Here's how the part is built. I have some questions about the finished solid (model axes, mm). A direction names the side the tool comes from. Give positions to 0.01 mm unless a question says otherwise; leave off trailing zeros. Loops run counter-clockwise (first coordinate to the right, second up) from the corner with the lowest first, then second, coordinate; pieces in that order, holes last. Notation, with made-up numbers: (59.25, 8.25) -> (96.25, 8.25) arc R9 ccw to (96.25, 18.25) -> close; hole circle Ø11 at (87, 54.5). An arc over 180 degrees is marked (long way). Answer in a Markdown table with one row per item. Add a question column.
Item 1: If we section it at D-D (x = 3.5): Write out the boundary of the cut face in (y, z).
Item 2: For P1, Ø6, axis at x = -4, z = -9.5, coming from the +Y side; P2, Ø2.5, axis at x = -0.5, z = 7, coming from the +Y side (3 decimals); P3, Ø4.5, axis at x = -1.5, z = 3, coming from the -Y side (3 decimals); P4, Ø1.9, axis at x = -0.5, y = -1.5, coming from the +Z side, each with a flat end and sliding along its axis, tell me the tip position at first contact or that it passes through.
Item 3: If we section it at A-A (y = 0): Write out the boundary of the cut face in (x, z) (3 decimals), then the cut area to 3 significant figures.
Item 4: Which directions (+Z, -Z, +X, -X, +Y, -Y) give clear straight access to the entire face, cutting with the end or side of a thin tool? Please do faces 1 (the face through (0, -4, 0)), 2 (the face through (-4.165, 0.051, 5.817)), 3 (the face through (0, -3.175, 6)), 4 (the face through (4.165, -0.051, 5.817)).
Item 5: If we section it at C-C (z = -19): Write out the boundary of the cut face in (x, y), then the cut area to 3 significant figures.
Item 6: If I drill on line 1 (Z direction, x = 2.75, y = -2.5); line 2 (Y direction, x = -1, z = 6) (3 decimals); line 3 (Z direction, x = 0.5, y = 1.5), over which ranges is the centre line in solid material (lowest first)?
Item 7: If we section it at B-B (x = 0): Write out the boundary of the cut face in (y, z) (3 decimals).
```python
from build123d import *

# Parameters (mm, degrees)
SKETCH002_R  = 1.7
PAD002_DEPTH = 5.8
SKETCH003_R  = 1.27
PAD003_DEPTH = 2.9
PAD_DEPTH    = 11.8
SKETCH001_R  = 5.58
PAD001_DEPTH = 32.15


with BuildPart() as metal:
    # Sketch002 → Pad002 (new body)
    with BuildSketch(Plane.XY):
        Circle(SKETCH002_R)
    extrude(amount=PAD002_DEPTH)

    # Sketch003 (on Face3 of Pad002) → Pad003 (join)
    with BuildSketch(Plane.XY.offset(5.8)):
        Circle(SKETCH003_R)
    extrude(amount=PAD003_DEPTH)


with BuildPart() as metal_1:
    # Body001 placement: moved
    add(metal.part.moved(Location((0, 0, 11.8))))


with BuildPart() as obj1:
    # Sketch → Pad (new body)
    with BuildSketch(Plane.XY):
        with BuildLine():
            ThreePointArc((-2.695663, 3.175), (-4.165, 0), (-2.695663, -3.175))
            Line((-2.695663, -3.175), (2.695663, -3.175))
            ThreePointArc((2.695663, -3.175), (4.165, 0), (2.695663, 3.175))
            Line((-2.695663, 3.175), (2.695663, 3.175))
        make_face()
    extrude(amount=PAD_DEPTH)

    # Sketch001 (on Sketch) → Pad001 (join)
    with BuildSketch(Plane.XY):
        Circle(SKETCH001_R)
    extrude(amount=-PAD001_DEPTH)

    # Fusion: union metal
    add(metal_1.part)


solid = obj1.part
```
Recorded:
| question | item | result |
|---|---|---|
| 1 | outline | (-4.35, -32.15) -> (4.35, -32.15) -> (4.35, 0) -> (2.26, 0) -> (2.26, 11.8) -> (-2.26, 11.8) -> (-2.26, 0) -> (-4.35, 0) -> close |
| 2 | P1 | stops at y = 5.49 |
| 2 | P2 | stops at y = 3.175 |
| 2 | P3 | stops at y = -3.175 |
| 2 | P4 | stops at z = 20.5 |
| 3 | outline | (-5.58, -32.15) -> (5.58, -32.15) -> (5.58, 0) -> (4.165, 0) -> (4.165, 11.8) -> (1.7, 11.8) -> (1.7, 17.6) -> (1.27, 17.6) -> (1.27, 20.5) -> (-1.27, 20.5) -> (-1.27, 17.6) -> (-1.7, 17.6) -> (-1.7, 11.8) -> (-4.165, 11.8) -> (-4.165, 0) -> (-5.58, 0) -> close |
| 3 | area | 484 mm^2 |
| 4 | face 1 | +Z |
| 4 | face 2 | +Z, -X |
| 4 | face 3 | +Z, +X, -X, -Y |
| 4 | face 4 | +Z, +X |
| 5 | outline | circle Ø11.16 at (0, 0) |
| 5 | area | 97.8 mm^2 |
| 6 | line 1 | z = -32.15 to 11.8 |
| 6 | line 2 | y = -3.175 to 3.175 |
| 6 | line 3 | z = -32.15 to 17.6 |
| 7 | outline | (-5.58, -32.15) -> (5.58, -32.15) -> (5.58, 0) -> (3.175, 0) -> (3.175, 11.8) -> (1.7, 11.8) -> (1.7, 17.6) -> (1.27, 17.6) -> (1.27, 20.5) -> (-1.27, 20.5) -> (-1.27, 17.6) -> (-1.7, 17.6) -> (-1.7, 11.8) -> (-3.175, 11.8) -> (-3.175, 0) -> (-5.58, 0) -> close |
